Work out the finished part from the listing and answer in its coordinate system (mm). A direction names the side the tool comes from. Coordinates: 2 decimals unless noted, no trailing zeros. Loops run counter-clockwise (first coordinate to the right, second up) from the corner with the lowest first, then second, coordinate; pieces in that order, holes last. Notation, with made-up numbers: (30, -38) -> (35, -38) arc R21 ccw to (35, -24) -> close; hole circle Ø7 at (30.25, 3.25). An arc over 180 degrees is marked (long way). Use a Markdown table: item, result.
from build123d import *

# Parameters (mm, degrees)
SKETCH1_W                       = 113
SKETCH1_H                       = 85
BOSS_EXTRUDE1_DEPTH             = 4
BOSS_EXTRUDE3_REACH             = 72.813
SKETCH4_W                       = 16
SKETCH4_H                       = 16
BOSS_EXTRUDE3_DIRECTION_2_DEPTH = 1
SKETCH10_W                      = 10
SKETCH10_H                      = 16
BOSS_EXTRUDE6_DEPTH             = 4
SKETCH6_W                       = 73
SKETCH6_H                       = 45
SKETCH6_W_2                     = 15
SKETCH6_H_2                     = 85
SKETCH6_W_3                     = 66
SKETCH6_H_3                     = 8
CUT_EXTRUDE2_DEPTH              = 82.483127088
SKETCH8_R                       = 6.1
CUT_EXTRUDE3_DEPTH              = 3.2
SKETCH9_W                       = 16
SKETCH9_H                       = 16
SKETCH9_W_2                     = 14
SKETCH9_H_2                     = 14
BOSS_EXTRUDE5_DEPTH             = 3
FILLET1_R                       = 0.2
SKETCH13_W                      = 85
SKETCH13_H                      = 4
CUT_EXTRUDE4_DEPTH              = 5
SKETCH14_W                      = 93
SKETCH14_H                      = 45
CUT_EXTRUDE5_DEPTH              = 82.722090037
SKETCH15_W                      = 12
SKETCH15_H                      = 45
BOSS_EXTRUDE7_DEPTH             = 4
BOSS_EXTRUDE8_DEPTH             = 15
SKETCH17_W                      = 42
SKETCH17_H                      = 117
CUT_EXTRUDE6_DEPTH              = 15
SKETCH18_W                      = 8
SKETCH18_H                      = 45
BOSS_EXTRUDE9_DEPTH             = 4


with BuildPart() as part:
    # Sketch1 → Boss-Extrude1 (new body)
    with BuildSketch(Plane(origin=(0, 0, 0), x_dir=(1, 0, 0), z_dir=(0, 1, 0))):
        Rectangle(SKETCH1_W, SKETCH1_H)
    extrude(amount=BOSS_EXTRUDE1_DEPTH)

    # Boss-Extrude3: up to this face of the body (flat: up to its plane)
    boss_extrude3_end = Plane(part.part.faces().sort_by_distance((0, 4, 0))[0])
    # Sketch4 → Boss-Extrude3 (add, up to the picked face)
    with BuildSketch(Plane.XZ, mode=Mode.PRIVATE) as boss_extrude3_sk1:
        with Locations((-48.5, 50.5)):
            Rectangle(SKETCH4_W, SKETCH4_H)
    boss_extrude3_tool1 = split(extrude(boss_extrude3_sk1.sketch, amount=-BOSS_EXTRUDE3_REACH, mode=Mode.PRIVATE), bisect_by=boss_extrude3_end, keep=Keep.BOTH, mode=Mode.PRIVATE)
    # Sketch4 → Boss-Extrude3 (add, up to the picked face)
    with BuildSketch(Plane.XZ, mode=Mode.PRIVATE) as boss_extrude3_sk2:
        with Locations((43.5, 50.5)):
            Rectangle(SKETCH4_W, SKETCH4_H)
    boss_extrude3_tool2 = split(extrude(boss_extrude3_sk2.sketch, amount=-BOSS_EXTRUDE3_REACH, mode=Mode.PRIVATE), bisect_by=boss_extrude3_end, keep=Keep.BOTH, mode=Mode.PRIVATE)
    # Sketch4 → Boss-Extrude3 (add, up to the picked face)
    with BuildSketch(Plane.XZ, mode=Mode.PRIVATE) as boss_extrude3_sk3:
        with Locations((43.5, -50.5)):
            Rectangle(SKETCH4_W, SKETCH4_H)
    boss_extrude3_tool3 = split(extrude(boss_extrude3_sk3.sketch, amount=-BOSS_EXTRUDE3_REACH, mode=Mode.PRIVATE), bisect_by=boss_extrude3_end, keep=Keep.BOTH, mode=Mode.PRIVATE)
    # Sketch4 → Boss-Extrude3 (add, up to the picked face)
    with BuildSketch(Plane.XZ, mode=Mode.PRIVATE) as boss_extrude3_sk4:
        with Locations((-48.5, -50.5)):
            Rectangle(SKETCH4_W, SKETCH4_H)
    boss_extrude3_tool4 = split(extrude(boss_extrude3_sk4.sketch, amount=-BOSS_EXTRUDE3_REACH, mode=Mode.PRIVATE), bisect_by=boss_extrude3_end, keep=Keep.BOTH, mode=Mode.PRIVATE)
    add(boss_extrude3_tool1.solids().sort_by(Axis((-48.5, 0, 50.5), (0, 1, 0)))[0])
    add(boss_extrude3_tool2.solids().sort_by(Axis((43.5, 0, 50.5), (0, 1, 0)))[0])
    add(boss_extrude3_tool3.solids().sort_by(Axis((43.5, 0, -50.5), (0, 1, 0)))[0])
    add(boss_extrude3_tool4.solids().sort_by(Axis((-48.5, 0, -50.5), (0, 1, 0)))[0])

    # Sketch4 → Boss-Extrude3 direction 2 (add)
    with BuildSketch(Plane.XZ):
        with Locations((-48.5, 50.5)):
            Rectangle(SKETCH4_W, SKETCH4_H)
        with Locations((43.5, 50.5)):
            Rectangle(SKETCH4_W, SKETCH4_H)
        with Locations((43.5, -50.5)):
            Rectangle(SKETCH4_W, SKETCH4_H)
        with Locations((-48.5, -50.5)):
            Rectangle(SKETCH4_W, SKETCH4_H)
    extrude(amount=BOSS_EXTRUDE3_DIRECTION_2_DEPTH)

    # Sketch10 → Boss-Extrude6 (add)
    with BuildSketch(Plane(origin=(0, 4, 0), x_dir=(1, 0, 0), z_dir=(0, 1, 0))):
        with Locations((-35.5, -50.5)):
            Rectangle(SKETCH10_W, SKETCH10_H)
        with Locations((-35.5, 50.5)):
            Rectangle(SKETCH10_W, SKETCH10_H)
    extrude(amount=-BOSS_EXTRUDE6_DEPTH)

    # Sketch6 → Cut-Extrude2 (cut, through all)
    with BuildSketch(Plane(origin=(0, 4, 0), x_dir=(1, 0, 0), z_dir=(0, 1, 0))):
        with Locations((5, 0)):
            Rectangle(SKETCH6_W, SKETCH6_H)
        with Locations((-49, 0)):
            Rectangle(SKETCH6_W_2, SKETCH6_H_2)
        with Locations((2.5, 38.5)):
            Rectangle(SKETCH6_W_3, SKETCH6_H_3)
        with Locations((2.5, -38.5)):
            Rectangle(SKETCH6_W_3, SKETCH6_H_3)
    extrude(amount=-CUT_EXTRUDE2_DEPTH, mode=Mode.SUBTRACT)

    # Sketch8 → Cut-Extrude3 (cut)
    with BuildSketch(Plane.XZ.offset(1)):
        with Locations(Location((-48.5, 50.5, 0), (0, 0, 270))):
            Circle(SKETCH8_R)
        with Locations(Location((43.5, 50.5, 0), (0, 0, 270))):
            Circle(SKETCH8_R)
        with Locations(Location((43.5, -50.5, 0), (0, 0, 90))):
            Circle(SKETCH8_R)
        with Locations(Location((-48.5, -50.5, 0), (0, 0, 90))):
            Circle(SKETCH8_R)
    extrude(amount=-CUT_EXTRUDE3_DEPTH, mode=Mode.SUBTRACT)

    # Sketch9 → Boss-Extrude5 (add)
    # profile 1 of 4: a face of its own
    with BuildSketch(Plane.XZ.offset(1)):
        with Locations((-48.5, 50.5)):
            Rectangle(SKETCH9_W, SKETCH9_H)
        with Locations((-48.5, 50.5)):
            Rectangle(SKETCH9_W_2, SKETCH9_H_2, mode=Mode.SUBTRACT)
    # profile 2 of 4: a face of its own
    with BuildSketch(Plane.XZ.offset(1)):
        with Locations((43.5, 50.5)):
            Rectangle(SKETCH9_W, SKETCH9_H)
        with Locations((43.5, 50.5)):
            Rectangle(SKETCH9_W_2, SKETCH9_H_2, mode=Mode.SUBTRACT)
    # profile 3 of 4: a face of its own
    with BuildSketch(Plane.XZ.offset(1)):
        with Locations((43.5, -50.5)):
            Rectangle(SKETCH9_W, SKETCH9_H)
        with Locations((43.5, -50.5)):
            Rectangle(SKETCH9_W_2, SKETCH9_H_2, mode=Mode.SUBTRACT)
    # profile 4 of 4: a face of its own
    with BuildSketch(Plane.XZ.offset(1)):
        with Locations((-48.5, -50.5)):
            Rectangle(SKETCH9_W, SKETCH9_H)
        with Locations((-48.5, -50.5)):
            Rectangle(SKETCH9_W_2, SKETCH9_H_2, mode=Mode.SUBTRACT)
    extrude(amount=BOSS_EXTRUDE5_DEPTH)

    # Fillet1
    fillet1_edges = [part.edges().sort_by_distance(p)[0] for p in [
        (-48.5, -1, -56.6),
        (43.5, -1, -56.6),
        (43.5, -1, 56.6),
        (-48.5, -1, 56.6),
    ]]
    fillet(fillet1_edges, radius=FILLET1_R)

    # Sketch13 → Cut-Extrude4 (cut)
    with BuildSketch(Plane(origin=(56.5, 0, 0), x_dir=(0, 0, -1), z_dir=(1, 0, 0))):
        with Locations((0, 2)):
            Rectangle(SKETCH13_W, SKETCH13_H)
    extrude(amount=-CUT_EXTRUDE4_DEPTH, mode=Mode.SUBTRACT)

    # Sketch14 → Cut-Extrude5 (cut, through all)
    with BuildSketch(Plane(origin=(0, 4, 0), x_dir=(1, 0, 0), z_dir=(0, 1, 0))):
        with Locations((5, 0)):
            Rectangle(SKETCH14_W, SKETCH14_H)
    extrude(amount=-CUT_EXTRUDE5_DEPTH, mode=Mode.SUBTRACT)


with BuildPart() as cut_extrude5_piece_1:
    # of the separate pieces the step leaves, piece 1, a body of its own (cut_extrude5_pieces)
    add(part.part.solids().sort_by_distance((-40.5, 0, -42.5))[0])



with BuildPart() as cut_extrude5_piece_2:
    # of the separate pieces the step leaves, piece 2, a body of its own (cut_extrude5_pieces)
    add(part.part.solids().sort_by_distance((-48.5, -1, 44.2))[0])


with BuildPart() as cut_extrude5_piece_1_1:
    add(cut_extrude5_piece_1.part)

    add(cut_extrude5_piece_2.part)  # Boss-Extrude7 merges Cut-Extrude5 piece 2
    # Sketch15 → Boss-Extrude7 (add)
    with BuildSketch(Plane(origin=(0, 4, 0), x_dir=(1, 0, 0), z_dir=(0, 1, 0))):
        with Locations((-12.5, 0)):
            Rectangle(SKETCH15_W, SKETCH15_H)
        with Locations((30.5, 0)):
            Rectangle(SKETCH15_W, SKETCH15_H)
    extrude(amount=-BOSS_EXTRUDE7_DEPTH)

    # Sketch16 → Boss-Extrude8 (add)
    with BuildSketch(Plane.XZ):
        Polygon((-6.5, -22.5), (-6.5, 22.5), (14.5, 22.5), (14.5, 34.5), (-30.5, 34.5), (-41.5, 34.5), (-41.5, 22.5), (-18.5, 22.5), (-18.5, -22.5), (-41.5, -22.5), (-41.5, -34.5), (-30.5, -34.5), (14.5, -34.5), (14.5, -22.5), align=None)
    extrude(amount=BOSS_EXTRUDE8_DEPTH)

    # Sketch17 → Cut-Extrude6 (cut)
    with BuildSketch(Plane(origin=(0, 4, 0), x_dir=(1, 0, 0), z_dir=(0, 1, 0))):
        with Locations((-12.5, 0)):
            Rectangle(SKETCH17_W, SKETCH17_H)
    extrude(amount=-CUT_EXTRUDE6_DEPTH, mode=Mode.SUBTRACT)

    # Sketch18 → Boss-Extrude9 (add)
    with BuildSketch(Plane(origin=(0, 4, 0), x_dir=(1, 0, 0), z_dir=(0, 1, 0))):
        with Locations((-37.5, 0)):
            Rectangle(SKETCH18_W, SKETCH18_H)
    extrude(amount=-BOSS_EXTRUDE9_DEPTH)


solid = cut_extrude5_piece_1_1.part
Q1. Section A-A on z = 10 is taken. Determine the outline of the cut face in (x, y), and give its area (3 significant figures).
Solved:
| item | result |
|---|---|
| outline | (-41.5, 0) -> (-33.5, 0) -> (-33.5, 4) -> (-41.5, 4) -> close; (-18.5, -15) -> (-6.5, -15) -> (-6.5, -11) -> (-18.5, -11) -> close; (24.5, 0) -> (36.5, 0) -> (36.5, 4) -> (24.5, 4) -> close |
| area | 128 mm² |
Q2. For faces 1 (the flat face through (-49, -2, 43.5)), 2 (the flat face through (-40.5, -2, -51)), 3 (the flat face through (44, 2, -22.5)), 4 (the flat face through (8.5, -3, -28)), determine the directions among +Z, -Z, +X, -X, +Y, -Y from which every point of the face is accessible in a straight line to the end or side of a thin tool.
Solved:
| item | result |
|---|---|
| face 1 | -Y |
| face 2 | -Z, -Y |
| face 3 | +X, +Y, -Y |
| face 4 | +Z, -Z, +Y |
Q3. Consider line 1 (X direction, y = -4.5, z = -27); line 2 (X direction, y = 0.35, z = 50.5); line 3 (Z direction, x = -49, y = 3). Determine where each line is inside the solid, lowest interval first. Write a range as [from, to].
Solved:
| item | result |
|---|---|
| line 1 | [-41.5, -33.5], [8.5, 14.5] |
| line 2 | [-56.5, -54.6], [-42.4, -33.5], [35.5, 37.4], [49.6, 51.5] |
| line 3 | [-58.5, -42.5], [42.5, 58.5] |
Q4. Given pin 1 Ø8 at (x, z) = (-46.5, -51) entering from -Y; pin 2 Ø3.5 at (y, z) = (-2.5, -31) entering from -X; pin 3 Ø10 at (x, y) = (23, -1) entering from +Z, each flat-ended and moving along its own axis, determine where each tip first touches the part or whether it passes through.
Solved:
| item | result |
|---|---|
| pin 1 | y = 2.2 |
| pin 2 | x = -41.5 |
| pin 3 | z = 34.5 |
Q5. Section B-B on x = -32 is taken. Determine the outline of the cut face in (y, z).
Solved:
| item | result |
|---|---|
| outline | (-15, -34.5) -> (-11, -34.5) -> (-11, -22.5) -> (-15, -22.5) -> close; (-15, 22.5) -> (-11, 22.5) -> (-11, 34.5) -> (-15, 34.5) -> close |
Q6. Determine the mould class of faces 5 (the flat face through (50.5, -2, -51)), 6 (the flat face through (51.5, 1, -45)), 7 (the flat face through (43, -2, 57.5)), 8 (the flat face through (43, 0, -58.5)) for opening direction X: pulls with the +X half, pulls with the -X half, needs draft (parallel to the pull), parting line crosses it, or undercut.
Solved:
| item | result |
|---|---|
| face 5 | undercut |
| face 6 | pulls with the +X half |
| face 7 | undercut |
| face 8 | needs draft |
Q7. Section C-C on z = 41 is taken. Determine the outline of the cut face in (x, y), and give its area (3 significant figures).
Solved:
| item | result |
|---|---|
| outline | (-41.5, 0) -> (-33.5, 0) -> (-33.5, 4) -> (-41.5, 4) -> close; (35.5, 0) -> (51.5, 0) -> (51.5, 4) -> (35.5, 4) -> close |
| area | 96.0 mm² |
Q8. Section D-D on x = -48.5 is taken. Determine the outline of the cut face in (y, z), and give its area (3 significant figures).
Solved:
| item | result |
|---|---|
| outline | (-4, -58.5) -> (4, -58.5) -> (4, -42.5) -> (-4, -42.5) -> (-4, -43.5) -> (-1, -43.5) -> (-1, -44.2) arc R0.2 ccw to (-0.8, -44.4) -> (2.2, -44.4) -> (2.2, -56.6) -> (-0.8, -56.6) arc R0.2 ccw to (-1, -56.8) -> (-1, -57.5) -> (-4, -57.5) -> close; (-4, 42.5) -> (4, 42.5) -> (4, 58.5) -> (-4, 58.5) -> (-4, 57.5) -> (-1, 57.5) -> (-1, 56.8) arc R0.2 ccw to (-0.8, 56.6) -> (2.2, 56.6) -> (2.2, 44.4) -> (-0.8, 44.4) arc R0.2 ccw to (-1, 44.2) -> (-1, 43.5) -> (-4, 43.5) -> close |
| area | 93.9 mm² |
